Work out the finished part from the listing and answer in its coordinate system (mm). Give positions to 0.01 mm unless a question says otherwise; leave off trailing zeros. Loops run counter-clockwise (first coordinate to the right, second up) from the corner with the lowest first, then second, coordinate; pieces in that order, holes last. Notation, with made-up numbers: M 15.5,-22.5 L 60.5,-22.5 A28 ccw 60.5,3.5 Z; hole C -34,33.25 d11. An arc over 180 degrees is marked long. Write item = value, one per line. Start each with the question number.
1. A flat-ended cylindrical pin translates along its axis: pin 1 Ø2.5 at (x, y) = (2.55, -39.5) entering from +Z. Find the tip coordinate at first contact, or state that the pin passes through.
2. The mould has two halves that part along Y. Classify faces 1 (the face through (2.225, -40.964, 1.014)), 2 (the face through (39, 0, 1)), 3 (the face through (39, -41, 2)): released by +Y, released by -Y, zero draft, split by the parting line, or undercut.
3. Section B-B on x = 76.95 is taken. Determine the outline of the cut face in (y, z), plus the area to 3 significant figures.
4. Section A-A on y = -2.7 is taken. Determine the outline of the cut face in (x, z), plus the area to 3 significant figures.
5. Consider L1, parallel to Y at x = 2.55, z = 0.6; L2, parallel to Y at x = 71.75, z = 1.55. Determine where each line is inside the solid, lowest interval first. Write a range as [from, to].
6. Section C-C on y = -79.5 is taken. Determine the outline of the cut face in (x, z).
```python
from build123d import *

# Parameters (mm, degrees)
SKETCH_1_W          = 79.5
SKETCH_1_H          = 83
EXTRUDE_1_DEPTH     = 2
SKETCH_2_R          = 1.5
SKETCH_2_R_2        = 1.65
CUT_EXTRUDE_1_DEPTH = 3
CUT_EXTRUDE_2_REACH = 116.949
SKETCH_3_R          = 1.6


with BuildPart() as part:
    # 草图1 → 凸台-拉伸1 (new body)
    with BuildSketch(Plane.XY):
        with Locations((39.75, -41.5)):
            Rectangle(SKETCH_1_W, SKETCH_1_H)
    extrude(amount=EXTRUDE_1_DEPTH)

    # 草图2 → 切除-拉伸1 (cut)
    with BuildSketch(Plane.XY.offset(2)):
        with Locations((2.55, -79.5)):
            Circle(SKETCH_2_R)
        with Locations((2.55, -39.5)):
            Circle(SKETCH_2_R)
        with Locations((76.95, -39.5)):
            Circle(SKETCH_2_R)
        with Locations((76.95, -79.5)):
            Circle(SKETCH_2_R)
        with Locations((2.55, -2.7)):
            Circle(SKETCH_2_R_2)
        with Locations(Location((76.95, -2.7, 0), (0, 0, 180))):
            Circle(SKETCH_2_R_2)
    extrude(amount=-CUT_EXTRUDE_1_DEPTH, mode=Mode.SUBTRACT)

    # 草图3 → 切除-拉伸2 (cut, up to next)
    with BuildSketch(Plane.XY, mode=Mode.PRIVATE) as cut_extrude_2_sk1:
        with Locations(Location((7.75, -30, 0), (0, 0, 180))):
            Circle(SKETCH_3_R)
    cut_extrude_2_tool1 = extrude(cut_extrude_2_sk1.sketch, amount=CUT_EXTRUDE_2_REACH, mode=Mode.PRIVATE) & part.part
    # 草图3 → 切除-拉伸2 (cut, up to next)
    with BuildSketch(Plane.XY, mode=Mode.PRIVATE) as cut_extrude_2_sk2:
        with Locations(Location((71.75, -30, 0), (0, 0, 180))):
            Circle(SKETCH_3_R)
    cut_extrude_2_tool2 = extrude(cut_extrude_2_sk2.sketch, amount=CUT_EXTRUDE_2_REACH, mode=Mode.PRIVATE) & part.part
    add(cut_extrude_2_tool1.solids().sort_by_distance((7.75, -30, 0))[0], mode=Mode.SUBTRACT)
    add(cut_extrude_2_tool2.solids().sort_by_distance((71.75, -30, 0))[0], mode=Mode.SUBTRACT)


solid = part.part
```
Verdict:
q1.pin_1 = through
q2.face_1 = undercut
q2.face_2 = released by +Y
q2.face_3 = zero draft
q3.outline = M -83,0 L -81,0 L -81,2 L -83,2 Z; M -78,0 L -41,0 L -41,2 L -78,2 Z; M -38,0 L -4.35,0 L -4.35,2 L -38,2 Z; M -1.05,0 L 0,0 L 0,2 L -1.05,2 Z
q3.area = 147 mm2
q4.outline = M 0,0 L 0.9,0 L 0.9,2 L 0,2 Z; M 4.2,0 L 75.3,0 L 75.3,2 L 4.2,2 Z; M 78.6,0 L 79.5,0 L 79.5,2 L 78.6,2 Z
q4.area = 146 mm2
q5.L1 = [-83, -81], [-78, -41], [-38, -4.35], [-1.05, 0]
q5.L2 = [-83, -31.6], [-28.4, 0]
q6.outline = M 0,0 L 1.05,0 L 1.05,2 L 0,2 Z; M 4.05,0 L 75.45,0 L 75.45,2 L 4.05,2 Z; M 78.45,0 L 79.5,0 L 79.5,2 L 78.45,2 Z
